```python
from build123d import *

# Parameters (mm, degrees)
F0_W     = 14
F0_H     = 15
F1_DEPTH = 4
F3_DEPTH = 15.001
F4_W     = 14
F4_H     = 6
F5_DEPTH = 2


with BuildPart() as f1:
    # F0 (on Top) → F1 (new body)
    with BuildSketch(Plane.XY):
        with Locations((0, 7.5)):
            Rectangle(F0_W, F0_H)
        with BuildLine():
            Line((-5, 4.9), (-5, 6.5))
            ThreePointArc((-5, 6.5), (-4, 7.5), (-3, 6.5))
            Line((-3, 6.5), (-3, 4.9))
            ThreePointArc((-3, 4.9), (-4, 3.9), (-5, 4.9))
        make_face(mode=Mode.SUBTRACT)
        with BuildLine():
            Line((5, 6.5), (5, 4.9))
            ThreePointArc((5, 4.9), (4, 3.9), (3, 4.9))
            Line((3, 4.9), (3, 6.5))
            ThreePointArc((3, 6.5), (4, 7.5), (5, 6.5))
        make_face(mode=Mode.SUBTRACT)
        with BuildLine():
            Line((-5, 10.9), (-5, 12.5))
            ThreePointArc((-5, 12.5), (-4, 13.5), (-3, 12.5))
            Line((-3, 12.5), (-3, 10.9))
            ThreePointArc((-3, 10.9), (-4, 9.9), (-5, 10.9))
        make_face(mode=Mode.SUBTRACT)
        with BuildLine():
            Line((3, 10.9), (3, 12.5))
            ThreePointArc((3, 12.5), (4, 13.5), (5, 12.5))
            Line((5, 12.5), (5, 10.9))
            ThreePointArc((5, 10.9), (4, 9.9), (3, 10.9))
        make_face(mode=Mode.SUBTRACT)
    extrude(amount=F1_DEPTH)

    # F2 (on face) → F3 (cut, through all)
    with BuildSketch(Plane.XZ):
        with BuildLine():
            ThreePointArc((2.75, 5), (2.702525, 4.491216), (2.561738, 4))
            Line((2.561738, 4), (2.75, 4))
            Line((2.75, 4), (2.75, 5))
        make_face()
        with BuildLine():
            Line((2.561738, 4), (-2.561738, 4))
            ThreePointArc((-2.561738, 4), (0, 2.25), (2.561738, 4))
        make_face()
        with BuildLine():
            ThreePointArc((-2.561738, 4), (-2.702525, 4.491216), (-2.75, 5))
            Line((-2.75, 5), (-2.75, 4))
            Line((-2.75, 4), (-2.561738, 4))
        make_face()
    extrude(amount=-F3_DEPTH, mode=Mode.SUBTRACT)

    # F4 (on face) → F5 (join)
    with BuildSketch(Plane(origin=(0, 0, 0), x_dir=(1, 0, 0), z_dir=(0, 0, -1))):
        with Locations((0, -12)):
            Rectangle(F4_W, F4_H)
        with BuildLine():
            ThreePointArc((-3, -12.5), (-4, -13.5), (-5, -12.5))
            Line((-5, -12.5), (-5, -10.9))
            ThreePointArc((-5, -10.9), (-4, -9.9), (-3, -10.9))
            Line((-3, -10.9), (-3, -12.5))
        make_face(mode=Mode.SUBTRACT)
        with BuildLine():
            ThreePointArc((5, -12.5), (4, -13.5), (3, -12.5))
            Line((3, -12.5), (3, -10.9))
            ThreePointArc((3, -10.9), (4, -9.9), (5, -10.9))
            Line((5, -10.9), (5, -12.5))
        make_face(mode=Mode.SUBTRACT)
    extrude(amount=F5_DEPTH)


solid = f1.part
```
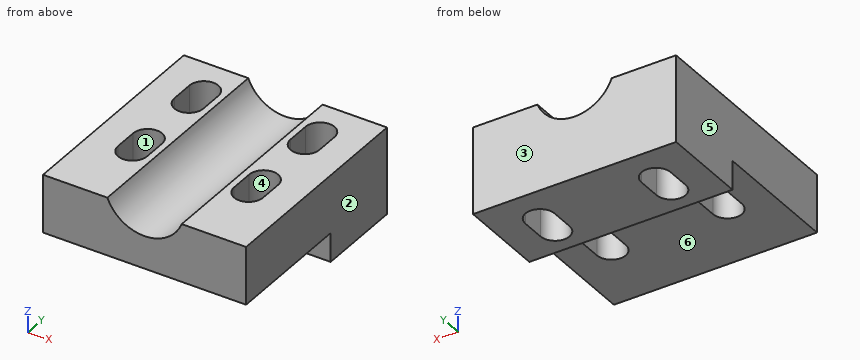
Source: CAD feature listing. Evaluate the final solid. Frame: model axes, mm. Face numbers are marked on the shaded views. A direction names the side the tool comes from. Coordinates: 2 decimals unless noted, no trailing zeros. Order: outer loops, then holes, each group sorted by start corner. A loop starts at its lowest first (then second) coordinate and runs counter-clockwise, first axis right, second up. Notation, with made-up numbers: M -16.75,-35 L 14.25,-35 A18 ccw 14.25,-14 Z; hole C 59.5,54 d4. An arc over 180 degrees is marked long. Write each question's results on one line, items separated by ' | '. Start each with the question number.
1) Section query D-D (x = -5.75). Return the cut outline in (y, z).
2) Line query: line 1 (Y direction, x = -4, z = 0.8); line 2 (X direction, y = 12, z = -1.25); line 3 (X direction, y = 5.75, z = 2.75). Output: solid intervals per line, ascending. Write a range as from..to.
3) Contact query for a flat-ended pin moving along its axis: pin 1 Ø7 at (x, y) = (-2, 3) entering from -Z. Output: stop coordinate, or through.
4) Section query A-A (z = 3.2). Return the cut outline in (x, y), plus the area to 3 significant figures.
5) Section query B-B (x = 4). Return the cut outline in (y, z).
6) Draft query along X for the marked faces 1, 2 and 3. Return one class per face: released by +X, released by -X, zero draft, split by the parting line, or undercut.
7) Section query C-C (z = 1.15). Return the cut outline in (x, y), plus the area to 3 significant figures.
8) Access query for the marked faces 4, 5 and 6. Directions: +Z, -Z, +X, -X, +Y, -Y. A direction counts if a zero-diameter tool reaches every point of the face in a straight line with its end or side. Return the directions, or none.
Answers:
1) outline: M 0,0 L 9,0 L 9,-2 L 15,-2 L 15,4 L 0,4 Z
2) line 1: y = 0..3.9, 7.5..9.9, 13.5..15 | line 2: x = -7..-5, -3..3, 5..7 | line 3: x = -7..-5, -3..-1.58, 1.58..3, 5..7
3) pin 1: stops at z = 0
4) outline: M -7,0 L -2.08,0 L -2.08,15 L -7,15 Z; M 2.08,0 L 7,0 L 7,15 L 2.08,15 Z; hole M -5,4.9 A1 ccw -3,4.9 L -3,6.5 A1 ccw -5,6.5 Z; hole M -5,10.9 A1 ccw -3,10.9 L -3,12.5 A1 ccw -5,12.5 Z; hole M 3,4.9 A1 ccw 5,4.9 L 5,6.5 A1 ccw 3,6.5 Z; hole M 3,10.9 A1 ccw 5,10.9 L 5,12.5 A1 ccw 3,12.5 Z | area: 122 mm^2
5) outline: M 0,0 L 3.9,0 L 3.9,4 L 0,4 Z; M 7.5,0 L 9,0 L 9,-2 L 9.9,-2 L 9.9,4 L 7.5,4 Z; M 13.5,-2 L 15,-2 L 15,4 L 13.5,4 Z
6) face 1: undercut | face 2: released by +X | face 3: zero draft
7) outline: M -7,0 L 7,0 L 7,15 L -7,15 Z; hole M -5,4.9 A1 ccw -3,4.9 L -3,6.5 A1 ccw -5,6.5 Z; hole M -5,10.9 A1 ccw -3,10.9 L -3,12.5 A1 ccw -5,12.5 Z; hole M 3,4.9 A1 ccw 5,4.9 L 5,6.5 A1 ccw 3,6.5 Z; hole M 3,10.9 A1 ccw 5,10.9 L 5,12.5 A1 ccw 3,12.5 Z | area: 185 mm^2
8) face 4: +Z, -Z | face 5: +Z, -Z, -X, +Y, -Y | face 6: -Z, +X, -X, -Y
